The drawing under review shows one solid part. Ordinate dimensions are in mm from its lowest x, y, z. Round coordinates to 2 decimals unless told otherwise and drop trailing zeros. Order: outer loops, then holes, each group sorted by start corner. A loop starts at its lowest first (then second) coordinate and runs counter-clockwise, first axis right, second up. Notation, with made-up numbers: (49, 78) -> (90, 78) arc R19 cw to (90, 107) -> close; hole circle Ø11 at (-32.75, 38). An arc over 180 degrees is marked (long way). Use a Markdown table: item, result. Add a question column.
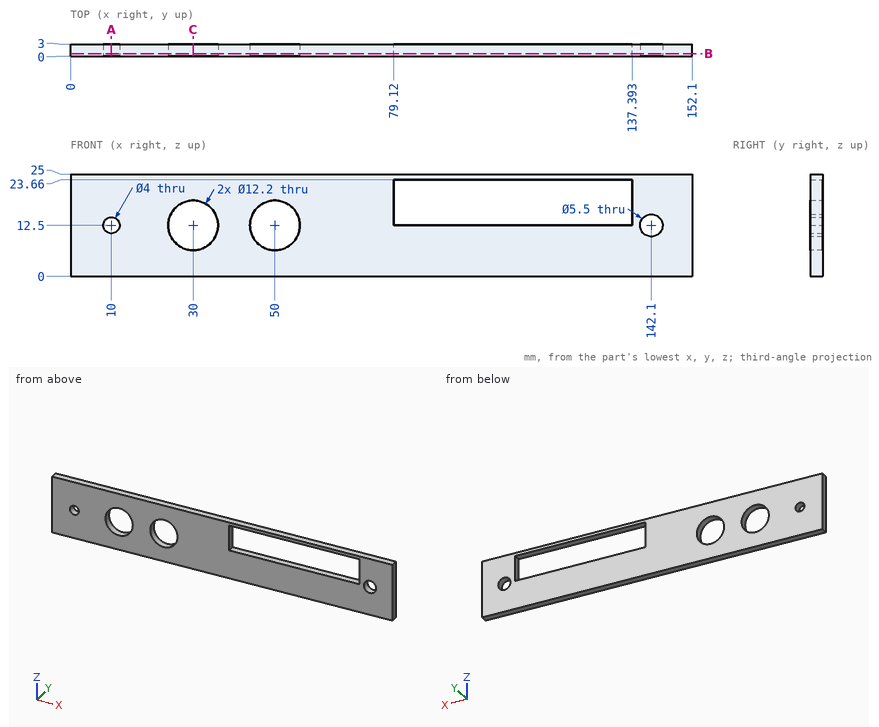
Q1. Add section C-C, the plane x = 30. Give the boundary of the cut face in (y, z).
Q2. To check wall thickness, follow line 1 along X through (y, z) = (2.5, 12.25) (1 decimal); line 2 along X through (y, z) = (2.05, 21); line 3 along X through (y, z) = (0.75, 17.5) (1 decimal). State the ranges of each line that lie inside material, in increasing order.
Q3. Add section A-A, the plane x = 10. Give the boundary of the cut face in (y, z), then the cut area to 3 significant figures.
Q4. For pin 1 (5 mm diameter, centred on x = 10, z = 12.5, fed in from +Y); pin 2 (3.5 mm diameter, centred on x = 142.1, z = 12.5, fed in from -Y), all flat-tipped, find the tip position at first contact; note any pin that passes through.
Q5. Add section B-B, the plane y = 0.65. Give the boundary of the cut face in (x, z), then the cut area to 3 significant figures.
Return value:
| question | item | result |
|---|---|---|
| 1 | outline | (0, 0) -> (3, 0) -> (3, 6.4) -> (0, 6.4) -> close; (0, 18.6) -> (3, 18.6) -> (3, 25) -> (0, 25) -> close |
| 2 | line 1 | 0 to 8, 12 to 23.9, 36.1 to 43.9, 56.1 to 139.4, 144.8 to 152.1 |
| 2 | line 2 | 0 to 79.12, 137.39 to 152.1 |
| 2 | line 3 | 0 to 26.5, 33.5 to 46.5, 53.5 to 79.1, 137.4 to 152.1 |
| 3 | outline | (0, 0) -> (3, 0) -> (3, 10.5) -> (0, 10.5) -> close; (0, 14.5) -> (3, 14.5) -> (3, 25) -> (0, 25) -> close |
| 3 | area | 63.0 mm² |
| 4 | pin 1 | y = 3 |
| 4 | pin 2 | through |
| 5 | outline | (0, 0) -> (152.1, 0) -> (152.1, 25) -> (0, 25) -> close; hole circle Ø4 at (10, 12.5); hole circle Ø12.2 at (30, 12.5); hole circle Ø12.2 at (50, 12.5); hole (79.12, 12.5) -> (137.39, 12.5) -> (137.39, 23.66) -> (79.12, 23.66) -> close; hole circle Ø5.5 at (142.1, 12.5) |
| 5 | area | 2,880 mm² |
